```python
from build123d import *

# Parameters (mm, degrees)
BASE_DEPTH                 = 60
MOTOR_TRASEIRO_START       = -5
MOTOR_TRASEIRO_DEPTH       = 30
ESBO_O3_10_R               = 1.5
MOTOR_EIXO_DEPTH           = 25
PADR_OCIRCULAR1_COUNT      = 2
PADR_OCIRCULAR1_ANGLE      = 285
ESPELHAR3_START            = -5
ESPELHAR3_COPY_1_DEPTH     = 30
ESPELHAR3_COPY_2_SKETCH_R  = 1.5
ESPELHAR3_COPY_2_DEPTH     = 25
ESBO_O16_R                 = 13
CAPACITORES_DEPTH          = 45
CORTE_EXTRUS_O1_DEPTH      = 8
ESBO_O19_W                 = 50.5
ESBO_O19_H                 = 39.838709678
CORTE_EXTRUS_O2_DEPTH      = 131.973279718
CORTE_EXTRUS_O3_DEPTH      = 151.021417999
CORTE_EXTRUS_O3_DEPTH_BACK = 151.021417999
ESBO_O21_W                 = 20
ESBO_O21_H                 = 50
ESBO_O24_W                 = 20
ESBO_O24_H                 = 5
CORTE_EXTRUS_O6_DEPTH      = 158.318148985
ESBO_O25_R                 = 1.5
CORTE_EXTRUS_O7_DEPTH      = 10


with BuildPart() as part:
    # Esboço1 → Base (new body)
    with BuildSketch(Plane(origin=(0, 0, 0), x_dir=(1, 0, 0), z_dir=(0, 1, 0))):
        with BuildLine():
            Line((-70.813516723, -26.97289629), (-26.97289629, -70.813516723))
            Line((-26.97289629, -70.813516723), (-34.043964102, -77.884584535))
            ThreePointArc((-34.043964102, -77.884584535), (-11.094726339, -84.272813217), (12.725930358, -84.041957953))
            Line((12.725930358, -84.041957953), (7.725930358, -75.381703915))
            Line((7.725930358, -75.381703915), (61.419505392, -44.381703915))
            Line((61.419505392, -44.381703915), (66.419505392, -53.041957953))
            ThreePointArc((66.419505392, -53.041957953), (85, 0), (66.419505392, 53.041957953))
            Line((66.419505392, 53.041957953), (61.419505392, 44.381703915))
            Line((61.419505392, 44.381703915), (7.725930358, 75.381703915))
            Line((7.725930358, 75.381703915), (12.725930358, 84.041957953))
            ThreePointArc((12.725930358, 84.041957953), (-11.094726339, 84.272813217), (-34.043964102, 77.884584535))
            Line((-34.043964102, 77.884584535), (-26.97289629, 70.813516723))
            Line((-26.97289629, 70.813516723), (-70.813516723, 26.97289629))
            Line((-70.813516723, 26.97289629), (-77.884584535, 34.043964102))
            ThreePointArc((-77.884584535, 34.043964102), (-85, 0), (-77.884584535, -34.043964102))
            Line((-77.884584535, -34.043964102), (-70.813516723, -26.97289629))
        make_face()
    extrude(amount=BASE_DEPTH)

    # Esboço3 → Motor-traseiro (cut)
    with BuildSketch(Plane(origin=(-48.893206507, 0, 48.893206507), x_dir=(0.7071067811865515, 0, 0.7071067811865436), z_dir=(-0.7071067811865436, 0, 0.7071067811865515)).offset(MOTOR_TRASEIRO_START)):
        with BuildLine():
            ThreePointArc((-22.5, 25), (0, 2.5), (22.5, 25))
            Line((22.5, 25), (22.5, 80))
            Line((22.5, 80), (-22.5, 80))
            Line((-22.5, 80), (-22.5, 25))
        make_face()
    motor_traseiro = extrude(amount=-MOTOR_TRASEIRO_DEPTH, mode=Mode.SUBTRACT)

    # Esboço3<10> → Motor-eixo (cut)
    with BuildSketch(Plane(origin=(-48.893206507, 0, 48.893206507), x_dir=(0.7071067811865515, 0, 0.7071067811865436), z_dir=(-0.7071067811865436, 0, 0.7071067811865515))):
        with BuildLine():
            Line((2, 32.745966692), (2, 70))
            Line((2, 70), (-2, 70))
            Line((-2, 70), (-2, 32.745966692))
            ThreePointArc((-2, 32.745966692), (0, 17), (2, 32.745966692))
        make_face()
        with Locations((0, 14)):
            Circle(ESBO_O3_10_R)
        with Locations((-9.526279442, 30.5)):
            Circle(ESBO_O3_10_R)
        with Locations((9.526279442, 30.5)):
            Circle(ESBO_O3_10_R)
    motor_eixo = extrude(amount=-MOTOR_EIXO_DEPTH, mode=Mode.SUBTRACT)

    # PadrãoCircular1: Motor-traseiro, Motor-eixo ×2 about axis
    padr_ocircular1_axis = Axis((0, 60, 0), (0, -1, 0))
    add([motor_traseiro.rotate(padr_ocircular1_axis, i * PADR_OCIRCULAR1_ANGLE / (PADR_OCIRCULAR1_COUNT - 1)) for i in range(1, PADR_OCIRCULAR1_COUNT)], mode=Mode.SUBTRACT)
    add([motor_eixo.rotate(padr_ocircular1_axis, i * PADR_OCIRCULAR1_ANGLE / (PADR_OCIRCULAR1_COUNT - 1)) for i in range(1, PADR_OCIRCULAR1_COUNT)], mode=Mode.SUBTRACT)

    # Espelhar3: Motor-traseiro, Motor-eixo across plane
    add(motor_traseiro.mirror(Plane.XY), mode=Mode.SUBTRACT)
    add(motor_eixo.mirror(Plane.XY), mode=Mode.SUBTRACT)

    # Espelhar3 copy 1 sketch → Espelhar3 copy 1 (cut)
    with BuildSketch(Plane(origin=(34.572717875, 0, -59.881703915), x_dir=(0.8660254037844427, 0, 0.499999999999993), z_dir=(0.499999999999993, 0, -0.8660254037844427)).offset(ESPELHAR3_START)):
        with BuildLine():
            ThreePointArc((-22.5, -25), (0, -2.5), (22.5, -25))
            Line((22.5, -25), (22.5, -80))
            Line((22.5, -80), (-22.5, -80))
            Line((-22.5, -80), (-22.5, -25))
        make_face()
    extrude(amount=-ESPELHAR3_COPY_1_DEPTH, mode=Mode.SUBTRACT)

    # Espelhar3 copy 2 sketch → Espelhar3 copy 2 (cut)
    with BuildSketch(Plane(origin=(34.572717875, 0, -59.881703915), x_dir=(0.8660254037844427, 0, 0.499999999999993), z_dir=(0.499999999999993, 0, -0.8660254037844427))):
        with BuildLine():
            Line((2, -32.745966692), (2, -70))
            Line((2, -70), (-2, -70))
            Line((-2, -70), (-2, -32.745966692))
            ThreePointArc((-2, -32.745966692), (0, -17), (2, -32.745966692))
        make_face()
        with Locations((0, -14)):
            Circle(ESPELHAR3_COPY_2_SKETCH_R)
        with Locations((-9.526279442, -30.5)):
            Circle(ESPELHAR3_COPY_2_SKETCH_R)
        with Locations((9.526279442, -30.5)):
            Circle(ESPELHAR3_COPY_2_SKETCH_R)
    extrude(amount=-ESPELHAR3_COPY_2_DEPTH, mode=Mode.SUBTRACT)

    # Esboço16 → Capacitores (cut)
    with BuildSketch(Plane(origin=(0, 60, 0), x_dir=(1, 0, 0), z_dir=(0, 1, 0))):
        with Locations(Location((-8.22315011, -62.461026267, 0), (0, 0, 270))):
            Circle(ESBO_O16_R)
        with Locations(Location((-8.22315011, 62.461026267, 0), (0, 0, 270))):
            Circle(ESBO_O16_R)
    extrude(amount=-CAPACITORES_DEPTH, mode=Mode.SUBTRACT)

    # Esboço18 → Corte-extrusão1 (cut)
    with BuildSketch(Plane.XZ):
        Polygon((-33, -10), (-33, 10), (-8, 35), (0, 35), (40, 13), (40, -13), (0, -35), (-8, -35), align=None)
    extrude(amount=-CORTE_EXTRUS_O1_DEPTH, mode=Mode.SUBTRACT)

    # Esboço19 → Corte-extrusão2 (cut, through all)
    with BuildSketch(Plane.XZ.offset(-8)):
        with Locations((2.169354839, 0)):
            Rectangle(ESBO_O19_W, ESBO_O19_H)
    extrude(amount=-CORTE_EXTRUS_O2_DEPTH, mode=Mode.SUBTRACT)

    # Esboço21 → Corte-extrusão3 (cut, two sides: drawn at the far end of the back side and taken through both)
    with BuildSketch(Plane(origin=(-23.080645161, 0, 0), x_dir=(0, 0, -1), z_dir=(1, 0, 0)).offset(-CORTE_EXTRUS_O3_DEPTH_BACK)):
        with Locations((0, 33)):
            Rectangle(ESBO_O21_W, ESBO_O21_H)
    extrude(amount=CORTE_EXTRUS_O3_DEPTH + CORTE_EXTRUS_O3_DEPTH_BACK, mode=Mode.SUBTRACT)

    # Esboço24 → Corte-extrusão6 (cut, through all)
    with BuildSketch(Plane(origin=(-33, 0, 0), x_dir=(0, 0, -1), z_dir=(1, 0, 0))):
        with Locations((0, 5.5)):
            Rectangle(ESBO_O24_W, ESBO_O24_H)
    extrude(amount=-CORTE_EXTRUS_O6_DEPTH, mode=Mode.SUBTRACT)

    # Esboço25 → Corte-extrusão7 (cut)
    with BuildSketch(Plane.XZ.offset(-8)):
        with Locations(Location((-26.080645161, 13, 0), (0, 0, 270))):
            Circle(ESBO_O25_R)
        with Locations(Location((-10.080645161, 25.919354839, 0), (0, 0, 270))):
            Circle(ESBO_O25_R)
        with Locations(Location((5.419354839, 25.919354839, 0), (0, 0, 270))):
            Circle(ESBO_O25_R)
        with Locations(Location((30.419354839, 13, 0), (0, 0, 270))):
            Circle(ESBO_O25_R)
        with Locations(Location((30.419354839, -13, 0), (0, 0, 90))):
            Circle(ESBO_O25_R)
        with Locations(Location((5.419354839, -25.919354839, 0), (0, 0, 90))):
            Circle(ESBO_O25_R)
        with Locations(Location((-10.080645161, -25.919354839, 0), (0, 0, 90))):
            Circle(ESBO_O25_R)
        with Locations(Location((-26.080645161, -13, 0), (0, 0, 90))):
            Circle(ESBO_O25_R)
    extrude(amount=-CORTE_EXTRUS_O7_DEPTH, mode=Mode.SUBTRACT)


solid = part.part
```
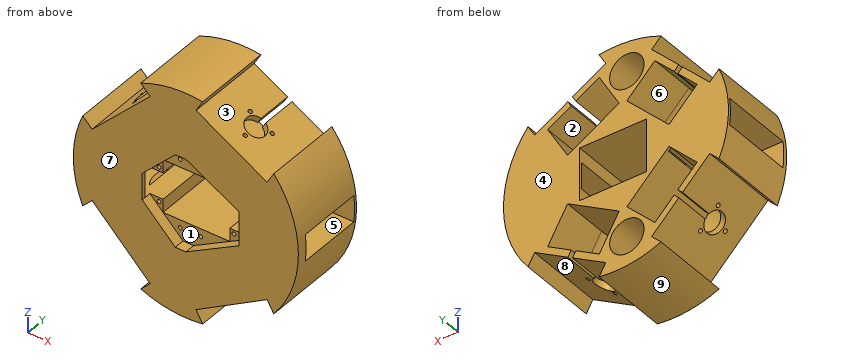
Can you work these out from the model? Positions are in its coordinate system, mm. Face numbers are marked on the shaded views. A direction names the side the tool comes from. Give positions to 0.01 mm unless a question says otherwise; leave off trailing zeros. Order: outer loops, then holes, each group sorted by start corner. A loop starts at its lowest first (then second) coordinate and runs counter-clockwise, first axis right, second up. Notation, with made-up numbers: (-31, 20.5) - (26, 20.5) arc R20 cw to (26, 53.5) - close; hole circle Ø7 at (4, 25.25). An arc over 180 degrees is marked (long way). Use a Markdown table: item, result. Add a question column.
Q1. If we section it at A-A on x = 75: Write out the boundary of the cut face in (y, z).
Q2. On a 3-axis mill with a long thin cutter (end or side, diameter ignored), from which of +Z, -Z, +X, -X, +Y, -Y can I reach the whole of each face in a straight line? I mean the marked faces 1, 2, 3, 4 and 5. Say none if no direction works.
Q3. If we section it at B-B on y = 23: Count the separate pieces of the cut face and the enclosed holes in it, plus the area to 3 significant figures.
Q4. I'm going to push flat-ended pins straight in: pin 1 (2.5 mm diameter, centred on x = -25.5, z = -12.5, fed in from -Y); pin 2 (8 mm diameter, centred on x = 33, y = 9, fed in from -Z); pin 3 (6 mm diameter, centred on x = -11, z = 14.5, fed in from -Y); pin 4 (1.5 mm diameter, centred on y = 1, z = 4.5, fed in from +X). Where does each tip first touch, or does it pass through?
Q5. Please list where these lines run through material, in increasing order: line 1 along X through (y, z) = (56.5, 40); line 2 along Z through (x, y) = (-26.5, 49); line 3 along X through (y, z) = (50.5, -16.5).
Q6. If we mould it in two halves opening along X, with no side actions, what happens to the marked faces 6, 7, 8 and 9? For each: released by +X, released by -X, zero draft, split by the parting line, or undercut.
Answers follow:
| question | item | result |
|---|---|---|
| 1 | outline | (0, -40) - (60, -40) - (60, 40) - (0, 40) - close; hole (8, -10) - (58, -10) - (58, 10) - (8, 10) - close |
| 2 | face 1 | -Y |
| 2 | face 2 | +Y |
| 2 | face 3 | +Y, -Y |
| 2 | face 4 | +Z, -Z, +X, -X, +Y |
| 2 | face 5 | +X, -X |
| 3 | separate pieces | 4 |
| 3 | enclosed holes | 2 |
| 3 | area | 8,100 mm^2 |
| 4 | pin 1 | stops at y = 8 |
| 4 | pin 2 | stops at z = -63.1 |
| 4 | pin 3 | passes through |
| 4 | pin 4 | stops at x = 84.92 |
| 5 | line 1 | x = -57.79 to -50.72, -8.29 to -0.99, 49.07 to 75 |
| 5 | line 2 | z = -80.76 to -58.32, -21.79 to -10, 10 to 21.79, 58.32 to 80.76 |
| 5 | line 3 | x = -83.38 to -48.32, -31.79 to -23.08, 27.42 to 83.38 |
| 6 | face 6 | undercut |
| 6 | face 7 | zero draft |
| 6 | face 8 | undercut |
| 6 | face 9 | split by the parting line |
